Design review of the part shown in the three views and the two pictorial views. Dimensions are in mm from the part's minimum x, y and z. Round coordinates to 2 decimals unless told otherwise and drop trailing zeros. Loops run counter-clockwise (first coordinate to the right, second up) from the corner with the lowest first, then second, coordinate; pieces in that order, holes last. Notation, with made-up numbers: M 30,13 L 84,13 A9 cw 84,25 Z; hole C 19.25,-28 d7. An arc over 180 degrees is marked long. Return JSON: item names as keys, results as strings. Group by question number.
Q1. To check wall thickness, follow line 1 along X through (y, z) = (198, 1.95); line 2 along X through (y, z) = (53, 2). State the ranges of each line that lie inside material, in increasing order.
Q2. Clearance check with flat-ended pins moving along their axes: pin 1 Ø0.8 at (y, z) = (120.5, 1.5) entering from +X; pin 2 Ø1.3 at (x, z) = (4.5, 1) entering from -Y; pin 3 Ø1.3 at (x, z) = (196, 1) entering from +Y. State where each tip first meets the part, or that it passes through.
Q3. Consider section B-B (y = 121). State the section outline as (x, z) points, and give its area (3 significant figures).
Q4. Consider section A-A (z = 1.25). State the section outline as (x, y) points.
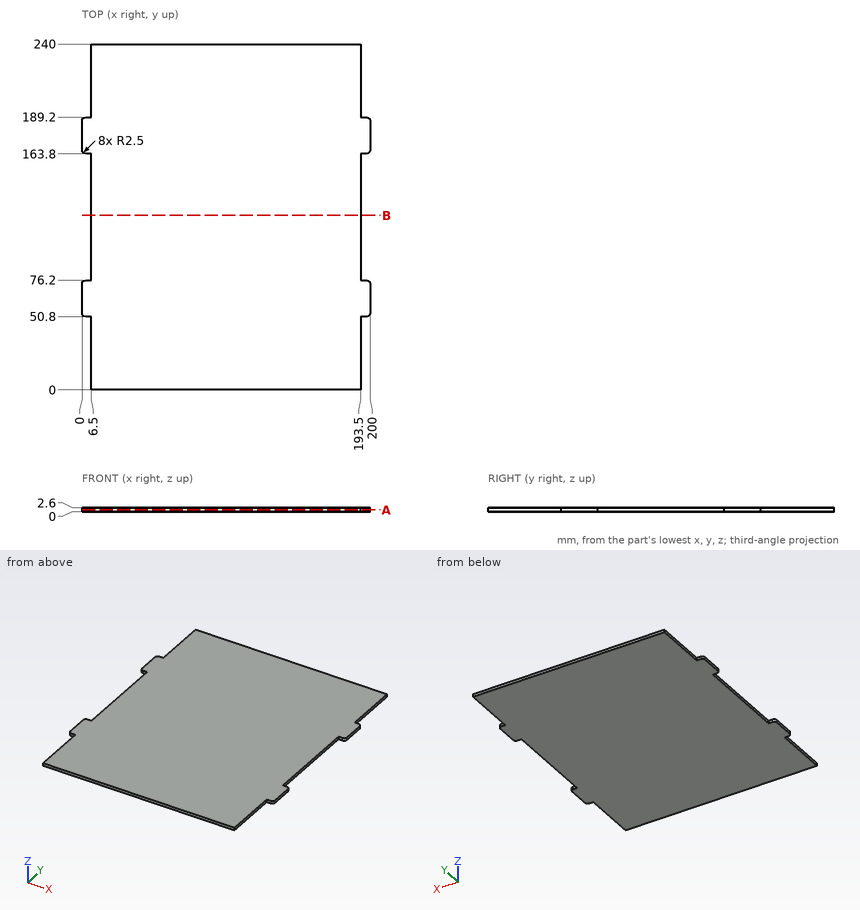
Values:
{
 "1": {"line 1": "x = 6.5 to 193.5", "line 2": "x = 0.02 to 199.98"},
 "2": {"pin 1": "stops at x = 193.5", "pin 2": "stops at y = 50.8", "pin 3": "stops at y = 189.2"},
 "3": {"outline": "M 6.5,0 L 193.5,0 L 193.5,2.6 L 6.5,2.6 Z", "area": "486 mm2"},
 "4": {"outline": "M 0,53.3 A2.5 ccw 2.5,50.8 L 6.5,50.8 L 6.5,0 L 193.5,0 L 193.5,50.8 L 197.5,50.8 A2.5 ccw 200,53.3 L 200,73.7 A2.5 ccw 197.5,76.2 L 193.5,76.2 L 193.5,163.8 L 197.5,163.8 A2.5 ccw 200,166.3 L 200,186.7 A2.5 ccw 197.5,189.2 L 193.5,189.2 L 193.5,240 L 6.5,240 L 6.5,189.2 L 2.5,189.2 A2.5 ccw 0,186.7 L 0,166.3 A2.5 ccw 2.5,163.8 L 6.5,163.8 L 6.5,76.2 L 2.5,76.2 A2.5 ccw 0,73.7 Z"}
}
